Autodesk Inventor part; units mm, degrees
ref_plane "YZ Plane" through (0, 0, 0) normal (1, 0, 0) x (0, 1, 0)
ref_plane "XZ Plane" through (0, 0, 0) normal (0, 1, 0) x (-1, 0, 0)
ref_plane "XY Plane" through (0, 0, 0) normal (0, 0, 1) x (1, 0, 0)
sketch "Skizze1" plane through (0, 0, 0) normal (0, 0, 1) x (1, 0, 0)
  line L0 (-29.8259, 0) -> (29.8259, 0) construction
  circle A0 centre (0, 0) radius 16.2 construction
  circle A1 centre (0, 16.2) radius 3.6
  circle A2 centre (14.0296, -8.1) radius 3.6
  circle A3 centre (-14.0296, -8.1) radius 3.6
  line L1 (0, 0) -> (-14.0296, -8.1) construction
  line L2 (0, 0) -> (14.0296, -8.1) construction
  circle A4 centre (0, 16.2) radius 2.6
  circle A5 centre (-14.0296, -8.1) radius 2.6
  circle A6 centre (14.0296, -8.1) radius 2.6
  arc A7 (4.8497, 19) -> (-4.8497, 19) centre (0, 16.2) ccw
  arc A8 (-18.8794, -5.3) -> (-14.0296, -13.7) centre (-14.0296, -8.1) ccw
  line L3 (14.0296, -13.7) -> (-14.0296, -13.7)
  line L4 (-18.8794, -5.3) -> (-4.8497, 19)
  line L5 (18.8794, -5.3) -> (4.8497, 19)
  arc A9 (14.0296, -13.7) -> (18.8794, -5.3) centre (14.0296, -8.1) ccw
  line L6 (0, 29.4) -> (0, -23.8) construction
  line L7 (0, 0) -> (0, 16.2) construction
  circle A10 centre (0, 0) radius 10
  dimension "d0" = 7.2
  dimension "d1" = 32.4
  dimension "d2" = 120
  dimension "d8" = 1
  dimension "d12" = 2
  dimension "d13" = 120
  dimension "d14" = 20
extrude "Extrusion1" add sketch "Skizze1" along normal blind 2 contours L5 A9 L3 A8 L4 A7
extrude "Extrusion3" add sketch "Skizze1" along normal blind 1.5 from surface at 2 contours A1 | A2 | A3 | L5 A9 L3 A8 L4 A7
equation "\"d13\" = d2"
properties part number "Rotor"
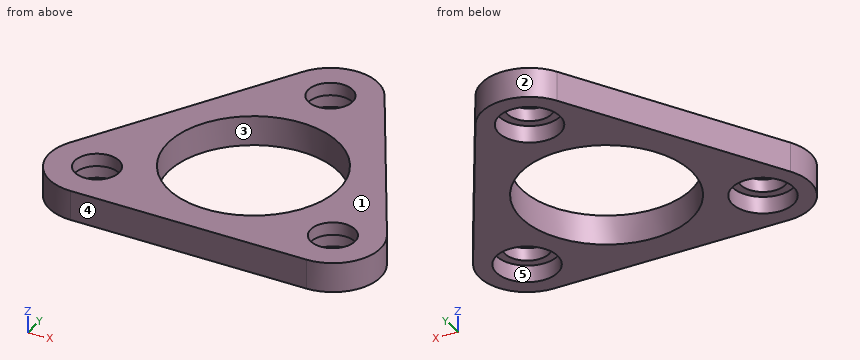
Could you check a few things on this model? Use its own coordinates, in mm. Face numbers are marked on the shaded views. A direction names the side the tool comes from. Give positions to 0.01 mm unless a question says otherwise; leave off trailing zeros. Order: outer loops, then holes, each group sorted by start corner. A loop starts at its lowest first (then second) coordinate and runs counter-clockwise, first axis right, second up. Notation, with made-up numbers: (54, 53.5) -> (106, 53.5) arc R25 cw to (106, 78.5) -> close; hole circle Ø11 at (58.25, 21.25). An arc over 180 degrees is marked (long way). Return JSON: item names as keys, results as strings.
1. Imagine slicing it at D-D on y = -8.1. List the corners of the cut face in (x, z) for me.
Answer list:
{"outline": "(-19.63, 0) -> (-17.63, 0) -> (-17.63, 2) -> (-16.63, 2) -> (-16.63, 3.5) -> (-19.63, 3.5) -> close; (-11.43, 2) -> (-10.43, 2) -> (-10.43, 0) -> (-5.86, 0) -> (-5.86, 3.5) -> (-11.43, 3.5) -> close; (5.86, 0) -> (10.43, 0) -> (10.43, 2) -> (11.43, 2) -> (11.43, 3.5) -> (5.86, 3.5) -> close; (16.63, 2) -> (17.63, 2) -> (17.63, 0) -> (19.63, 0) -> (19.63, 3.5) -> (16.63, 3.5) -> close"}
2. Imagine slicing it at C-C on y = 16.2. List the corners of the cut face in (x, z) for me.
Answer list:
{"outline": "(-6.47, 0) -> (-3.6, 0) -> (-3.6, 2) -> (-2.6, 2) -> (-2.6, 3.5) -> (-6.47, 3.5) -> close; (2.6, 2) -> (3.6, 2) -> (3.6, 0) -> (6.47, 0) -> (6.47, 3.5) -> (2.6, 3.5) -> close"}
3. For pin 1 Ø7 at (x, y) = (14.03, -8.1) entering from -Z; pin 2 Ø2 at (x, z) = (14, 3) entering from +Y, each with a flat end and sliding along its axis, tell me the tip position at first contact or that it passes through.
Answer list:
{"pin 1": "stops at z = 2", "pin 2": "stops at y = 4.88"}
4. On a 3-axis mill with a long thin cutter (end or side, diameter ignored), from which of +Z, -Z, +X, -X, +Y, -Y can I reach the whole of each face in a straight line? I mean the marked faces 4 and 5. Say none if no direction works.
Answer list:
{"face 4": "+Z, -Z, +X, -X, -Y", "face 5": "-Z"}
5. I need wall thicknesses on line 1 (Y direction, x = 0, z = 1); line 2 (Y direction, x = 0, z = 3.1); line 3 (X direction, y = -7.5, z = 1.5). Which ranges of each line are inside material? Lowest first, please. Write a range as from..to.
Answer list:
{"line 1": "y = -13.7..-10, 10..12.6, 19.8..21.8", "line 2": "y = -13.7..-10, 10..13.6, 18.8..21.8", "line 3": "x = -19.6..-17.58, -10.48..-6.61, 6.61..10.48, 17.58..19.6"}
6. Imagine slicing it at A-A on x = 0. List the corners of the cut face in (y, z) for me, then the cut area to 3 significant figures.
Answer list:
{"outline": "(-13.7, 0) -> (-10, 0) -> (-10, 3.5) -> (-13.7, 3.5) -> close; (10, 0) -> (12.6, 0) -> (12.6, 2) -> (13.6, 2) -> (13.6, 3.5) -> (10, 3.5) -> close; (18.8, 2) -> (19.8, 2) -> (19.8, 0) -> (21.8, 0) -> (21.8, 3.5) -> (18.8, 3.5) -> close", "area": "32.0 mm2"}
7. Imagine slicing it at B-B on z = 1.1. List the corners of the cut face in (x, y) for me.
Answer list:
{"outline": "(-18.88, -5.3) arc R5.6 ccw to (-14.03, -13.7) -> (14.03, -13.7) arc R5.6 ccw to (18.88, -5.3) -> (4.85, 19) arc R5.6 ccw to (-4.85, 19) -> close; hole circle Ø7.2 at (-14.03, -8.1); hole circle Ø20 at (0, 0); hole circle Ø7.2 at (0, 16.2); hole circle Ø7.2 at (14.03, -8.1)"}
8. Thinking about a two-plate mould opening in Y: for the marked faces 1, 2 and 3, which applies, pulls with the +Y half, pulls with the -Y half, needs draft (parallel to the pull), parting line crosses it, or undercut?
Answer list:
{"face 1": "needs draft", "face 2": "pulls with the +Y half", "face 3": "undercut"}
